Part model, mm, in its own coordinate system. A direction names the side the tool comes from. Coordinates: 2 decimals unless noted, no trailing zeros. Loops run counter-clockwise (first coordinate to the right, second up) from the corner with the lowest first, then second, coordinate; pieces in that order, holes last. Notation, with made-up numbers: M -27,-17.75 L 29,-17.75 A28 ccw 29,4.25 Z; hole C -9,75 d2. An arc over 180 degrees is marked long. Answer as a JSON object with one key per item and string values. Group by question number.
1. Drill centre lines: L1, parallel to Z at x = -2.5, y = 29.85; L2, parallel to X at y = 30, z = 5; L3, parallel to Z at x = -8, y = 30.4. Where is each one in solid material? Low to high.
2. 3-axis set-ups, long thin cutter, end or side, ignore diameter. For faces 1 (the face through (-9, 23, 1)), 2 (the face through (-2.53, 30.24, 4.25)), 3 (the face through (-5, -29.5, 7)), 4 (the face through (-3.19, -30.26, 4.65)): which of +Z, -Z, +X, -X, +Y, -Y reach the whole face in a straight line?
3. Mould opens along Z. For faces 5 (the face through (-5, 31, 5)), 6 (the face through (-6.67, 30.24, 5.69)), 7 (the face through (-4, 0, 10)) say: released by +Z, released by -Z, zero draft, split by the parting line, or undercut.
4. Saw through at C-C on x = -4.75. Write the cut outline in (y, z).
5. Drop flat-ended pins along their axis: pin 1 Ø1.6 at (x, z) = (-9, 9) entering from -Y; pin 2 Ø2 at (x, z) = (-2.5, 5) entering from +Y; pin 3 Ø4 at (y, z) = (-9.5, 5.5) entering from -X. Give the stop position or say it passes through.
6. Saw through at D-D on y = 26.5. Write the cut outline in (x, z), then the cut area to 3 significant figures.
7. Saw through at B-B on y = -13.5. Write the cut outline in (x, z), then the cut area to 3 significant figures.
8. Saw through at A-A on z = 5. Write the cut outline in (x, y), then the cut area to 3 significant figures.
Autodesk Inventor part; units mm, degrees
ref_plane "YZ Plane" through (0, 0, 0) normal (1, 0, 0) x (0, 1, 0)
ref_plane "XZ Plane" through (0, 0, 0) normal (0, 1, 0) x (-1, 0, 0)
ref_plane "XY Plane" through (0, 0, 0) normal (0, 0, 1) x (1, 0, 0)
sketch "Náčrt1" plane through (0, 0, 0) normal (0, 1, 0) x (-1, 0, 0)
  line L0 (0, -2) -> (0, 12)
  line L1 (-1.6, 0) -> (9.6, 0)
  line L2 (8, 10) -> (0, 10)
  line L3 (0, 10) -> (0, 0)
  line L4 (0, 0) -> (8, 0)
  line L5 (8, 0) -> (8, 10)
  line L6 (8, 8.5) -> (1.5, 8.5)
  line L7 (1.5, 8.5) -> (1.5, 1.5)
  line L8 (1.5, 1.5) -> (8, 1.5)
  line L9 (8, 1.5) -> (8, 8.5)
  point P0 (0, 0)
  point P1 (0, 10)
  dimension "d0" = 8
  dimension "d1" = 10
  dimension "d2" = 6.5
  dimension "d3" = 7
  dimension "d4" = 1.5
extrude "Vysunutí1" add sketch "Náčrt1" along normal mid plane 59 contours L0 L2 L5 L6 L7 L8 L1
sketch "Náčrt2" plane through (0, -29.5, 0) normal (0, -1, 0) x (1, 0, 0)
  line L0 (-8, 8.5) -> (-1.5, 8.5)
  line L1 (-1.5, 8.5) -> (-1.5, 1.5)
  line L2 (-1.5, 1.5) -> (-8, 1.5)
  line L3 (-8, 1.5) -> (-8, 0)
  line L4 (-8, 0) -> (0, 0)
  line L5 (0, 0) -> (0, 10)
  line L6 (0, 10) -> (-8, 10)
  line L7 (-8, 10) -> (-8, 8.5)
  line L8 (-8, 10) -> (0, 10)
  line L9 (0, 10) -> (0, 0)
  line L10 (0, 0) -> (-8, 0)
  line L11 (-8, 0) -> (-8, 10)
extrude "Vysunutí2" add sketch "Náčrt2" along normal blind 1.5
sketch "Náčrt3" plane through (0, -29.5, 0) normal (0, 1, 0) x (1, 0, 0)
  line L0 (-8, -8.5) -> (-1.5, -8.5)
  line L1 (-1.5, -8.5) -> (-1.5, -1.5)
  line L2 (-1.5, -1.5) -> (-8, -1.5)
  line L3 (-8, -8.5) -> (-8, -1.5)
  point P0 (0, 0)
  point P1 (-4.75, -5)
  dimension "d9" = 3.25
  dimension "d10" = 3.5
hole "Díra1" at (-4.75, -29.5, 5) direction (0, -1, 0) diameter 3.2 end through all
sketch "Náčrt5" plane through (0, 29.5, 0) normal (0, 1, 0) x (1, 0, 0)
  line L0 (0, -10) -> (-8, -10)
  line L1 (0, 0) -> (-8, 0)
  line L2 (-8, 0) -> (-8, -10)
  line L3 (-8, -10) -> (0, -10)
  line L4 (0, -10) -> (0, 0)
extrude "Vysunutí3" add sketch "Náčrt5" along normal blind 1.5
sketch "Náčrt6" plane through (-8, -31, 0) normal (-1, 0, 0) x (0, 0, 1)
  line L0 (0, 0) -> (0, 62)
  line L1 (0, 62) -> (0, 54)
  line L2 (0, 54) -> (1.5, 54)
  line L3 (1.5, 1.5) -> (1.5, 60.5)
  line L4 (1.5, 60.5) -> (1.5, 54)
  line L5 (0, 0) -> (0, 62)
  line L6 (10, 0) -> (0, 0)
  line L7 (10, 0) -> (10, 62)
  line L8 (0, 62) -> (10, 62)
  line L9 (1.5, 60.5) -> (8.5, 60.5)
  line L10 (8.5, 1.5) -> (8.5, 60.5)
  line L11 (8.5, 1.5) -> (1.5, 1.5)
  line L12 (1.5, 1.5) -> (1.5, 60.5)
  line L13 (1.5, 60.5) -> (8.5, 60.5)
  line L14 (8.5, 60.5) -> (8.5, 54)
  line L15 (8.5, 60.5) -> (8.5, 1.5)
  line L16 (10, 54) -> (8.5, 54)
  line L17 (10, 54) -> (10, 62)
  line L18 (0, 62) -> (10, 62)
  point P0 (0, 31)
  dimension "d31" = 8
  dimension "d32" = 8
extrude "Vysunutí4" add sketch "Náčrt6" along normal blind 3 contours L0 L8 L7 L16 L10 L9 L3 L2
sketch "Náčrt7" plane through (0, 31, 0) normal (0, 1, 0) x (1, 0, 0)
  line L0 (0, -10) -> (-11, -10)
  line L1 (0, -10) -> (0, 0)
  line L2 (0, 0) -> (-11, 0)
  line L3 (-11, -10) -> (-11, 0)
  point P0 (-2.5, -5)
  dimension "d35" = 2.5
  dimension "d37" = 5
hole "Díra3" at (-2.5, 31, 5) direction (0, -1, 0) diameter 1.5 depth 1.5
sketch "Náčrt8" plane through (0, 31, 0) normal (0, 1, 0) x (1, 0, 0)
  circle A0 centre (-2.5, -5) radius 0.75
  line L0 (0, -10) -> (-11, -10)
  line L1 (0, -10) -> (0, 0)
  line L2 (0, 0) -> (-11, 0)
  line L3 (-11, -10) -> (-11, 0)
  point P0 (-8, -5)
  dimension "d45" = 3
  dimension "d46" = 5
hole "Díra4" at (-8, 31, 5) direction (0, -1, 0) diameter 3 depth 1.5
properties part number "head_arm" material "Hliník 6061"
Outcome:
{
 "1": {"L1": "z = 0 to 4.25, 5.75 to 10", "L2": "x = -11 to -9.5, -6.5 to -3.25, -1.75 to 0", "L3": "z = 0 to 3.5, 6.5 to 10"},
 "2": {"face 1": "+Z, -Z, -X, -Y", "face 2": "+Y", "face 3": "-X", "face 4": "-Y"},
 "3": {"face 5": "zero draft", "face 6": "undercut", "face 7": "released by +Z"},
 "4": {"outline": "M -31,0 L 31,0 L 31,10 L -31,10 L -31,6.6 L -29.5,6.6 L -29.5,8.5 L 29.5,8.5 L 29.5,1.5 L -29.5,1.5 L -29.5,3.4 L -31,3.4 Z"},
 "5": {"pin 1": "stops at y = 23", "pin 2": "stops at y = 31", "pin 3": "stops at x = -1.5"},
 "6": {"outline": "M -11,0 L 0,0 L 0,10 L -11,10 L -11,8.5 L -1.5,8.5 L -1.5,1.5 L -11,1.5 Z", "area": "43.5 mm²"},
 "7": {"outline": "M -8,0 L 0,0 L 0,10 L -8,10 L -8,8.5 L -1.5,8.5 L -1.5,1.5 L -8,1.5 Z", "area": "34.5 mm²"},
 "8": {"outline": "M -11,29.5 L -9.5,29.5 L -9.5,31 L -11,31 Z; M -8,-31 L -6.35,-31 L -6.35,-29.5 L -8,-29.5 Z; M -6.5,29.5 L -3.25,29.5 L -3.25,31 L -6.5,31 Z; M -3.15,-31 L 0,-31 L 0,31 L -1.75,31 L -1.75,29.5 L -1.5,29.5 L -1.5,-29.5 L -3.15,-29.5 Z", "area": "105 mm²"}
}
